Here's how the part is built. I have some questions about the finished solid (model axes, mm). Face numbers are marked on the shaded views. A direction names the side the tool comes from. Round coordinates to 2 decimals unless told otherwise and drop trailing zeros. Order: outer loops, then holes, each group sorted by start corner. A loop starts at its lowest first (then second) coordinate and runs counter-clockwise, first axis right, second up. Notation, with made-up numbers: M 55,-6 L 92,-6 A24 cw 92,26 Z; hole C 24,-29 d2. An arc over 180 degrees is marked long. Write each question's results on one line, items separated by ' | '. Start each with the question number.
```python
from build123d import *

# Parameters (mm, degrees)
F1_DEPTH = 15
F3_D     = 6.6


with BuildPart() as f1:
    # F0 (on Front) → F1 (new body, symmetric)
    with BuildSketch(Plane.XZ):
        with BuildLine():
            ThreePointArc((1, 14.9666295471), (10.9544511501, 10.246950766), (15, 0))
            ThreePointArc((15, 0), (10.9544511501, -10.246950766), (1, -14.9666295471))
            Line((1, -14.9666295471), (1, -19.9666295471))
            Line((1, -19.9666295471), (2, -19.9666295471))
            Line((2, -19.9666295471), (2, -40))
            Line((2, -40), (20, -40))
            Line((20, -40), (20, 20))
            Line((20, 20), (1, 20))
            Line((1, 20), (1, 14.9666295471))
        make_face()
    extrude(amount=F1_DEPTH, both=True)

    # F3 (through all)
    with Locations(Plane(origin=(0, 0, 0), x_dir=(0, 1, 0), z_dir=(-1, 0, 0))):
        with Locations((0, 25)):
            Hole(F3_D / 2)


solid = f1.part
```
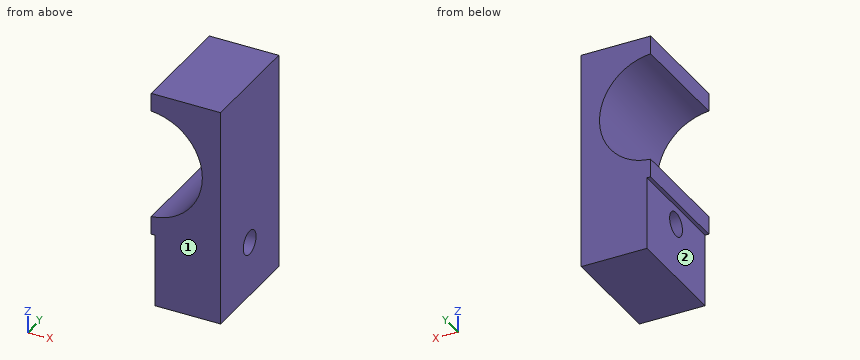
(1) On a 3-axis mill with a long thin cutter (end or side, diameter ignored), from which of +Z, -Z, +X, -X, +Y, -Y can I reach the whole of each face in a straight line? I mean the marked faces 1 and 2. Say none if no direction works.
(2) I'm going to push flat-ended pins straight in: pin 1 Ø16 at (y, z) = (0.5, -32) entering from -X; pin 2 Ø1 at (y, z) = (1.5, -6) entering from -X. Where does each tip first touch, or does it pass through?
(3) Please list where these lines run through material, in increasing order: line 1 (Z direction, x = 6.5, y = -1); line 2 (Y direction, x = 15, z = -25); line 3 (Z direction, x = 16, y = 0).
(4) I want a section at D-D on x = 9.5. Write out the boundary of the cut face in (y, z).
(5) I want a section at C-C on y = 0. Write out the boundary of the cut face in (x, z), and give its area (3 significant figures).
(6) I want a section at A-A on z = -25. Write out the boundary of the cut face in (x, y), and give its area (3 significant figures).
(7) I want a section at B-B on x = 4.5. Write out the boundary of the cut face in (y, z), and give its area (3 significant figures).
Solutions:
1) face 1: +Z, -Z, +X, -X, -Y | face 2: -Z, -X, +Y, -Y
2) pin 1: x = 2 | pin 2: x = 13.52
3) line 1: -40 to -28.14, -21.86 to -13.52, 13.52 to 20 | line 2: -15 to -3.3, 3.3 to 15 | line 3: -40 to -28.3, -21.7 to 20
4) outline: M -15,-40 L 15,-40 L 15,-11.61 L -15,-11.61 Z; M -15,11.61 L 15,11.61 L 15,20 L -15,20 Z; hole C 0,-25 d6.6
5) outline: M 1,-19.97 L 2,-19.97 L 2,-21.7 L 20,-21.7 L 20,20 L 1,20 L 1,14.97 A15 cw 1,-14.97 Z; M 2,-40 L 20,-40 L 20,-28.3 L 2,-28.3 Z | area: 678 mm^2
6) outline: M 2,-15 L 20,-15 L 20,-3.3 L 2,-3.3 Z; M 2,3.3 L 20,3.3 L 20,15 L 2,15 Z | area: 421 mm^2
7) outline: M -15,-40 L 15,-40 L 15,-14.31 L -15,-14.31 Z; M -15,14.31 L 15,14.31 L 15,20 L -15,20 Z; hole C 0,-25 d6.6 | area: 907 mm^2
